```python
from build123d import *

# Parameters (mm, degrees)
SKETCH_W        = 232
SKETCH_H        = 132
PAD_DEPTH       = 140
SKETCH001_W     = 200
SKETCH001_H     = 100
POCKET_DEPTH    = 130
SKETCH002_W     = 216
SKETCH002_H     = 116
SKETCH002_W_2   = 200
SKETCH002_H_2   = 100
PAD001_DEPTH    = 8
FILLET_R        = 5
SKETCH008_R     = 3.5
POCKET003_DEPTH = 16


with BuildPart() as part:
    # Sketch → Pad (new body)
    with BuildSketch(Plane.XY):
        Rectangle(SKETCH_W, SKETCH_H)
    extrude(amount=PAD_DEPTH)

    # Sketch001 (on Face6 of Pad) → Pocket (cut)
    with BuildSketch(Plane.XY.offset(140)):
        Rectangle(SKETCH001_W, SKETCH001_H)
    extrude(amount=-POCKET_DEPTH, mode=Mode.SUBTRACT)

    # Sketch002 (on Face5 of Pocket) → Pad001 (join)
    with BuildSketch(Plane.XY.offset(140)):
        Rectangle(SKETCH002_W, SKETCH002_H)
        Rectangle(SKETCH002_W_2, SKETCH002_H_2, mode=Mode.SUBTRACT)
    extrude(amount=PAD001_DEPTH)

    # Fillet
    fillet_edges = [part.edges().sort_by_distance(p)[0] for p in [
        (-116, -66, 70),
        (116, -66, 70),
        (116, 66, 70),
        (0, -66, 0),
        (116, 0, 0),
        (-100, 50, 79),
        (-100, -50, 79),
        (-116, 66, 70),
        (100, -50, 79),
        (100, 50, 79),
        (100, 0, 10),
        (0, -50, 10),
        (0, 50, 10),
        (-100, 0, 10),
        (108, -58, 144),
        (108, 58, 144),
        (-108, -58, 144),
        (-108, 58, 144),
        (0, 66, 0),
        (-116, 0, 0),
    ]]
    fillet(fillet_edges, radius=FILLET_R)

    # Sketch008 (on Face10 of Fillet) → Pocket003 (cut)
    with BuildSketch(Plane.YZ.offset(116)):
        with Locations((25, 19.8)):
            Circle(SKETCH008_R)
    extrude(amount=-POCKET003_DEPTH, mode=Mode.SUBTRACT)


solid = part.part
```
CAD build for the part. Positions are in the model's coordinates, mm. A direction names the side the tool comes from. Coordinates: 2 decimals unless noted, no trailing zeros. Write each loop counter-clockwise with the first axis right and the second up, starting at its lowest first coordinate (ties: lowest second). Pieces come first, ordered by that corner, then holes. Notation, with made-up numbers: (53, 6) -> (68, 6) arc R12 ccw to (68, 15) -> close; hole circle Ø5 at (81.5, 7.5). An arc over 180 degrees is marked (long way). Return JSON: item names as keys, results as strings. Group by question number.
Q1. Cut at A-A, the plane y = 25. Give the cut face in (x, z).
Q2. Cut at C-C, the plane z = 84. Give the cut face in (x, y).
Q3. Flat gauge pins, fed straight in: pin 1 (6 mm diameter, centred on x = 18, y = 26.5, fed in from +Z); pin 2 (4 mm diameter, centred on y = 12, z = 142.5, fed in from +X). Where does each tip first touch, or does it go through?
Q4. Cut at D-D, the plane z = 19.8. Give the cut face in (x, y), then the cut area to 3 significant figures.
Q5. Which spindle directions (+Z, -Z, +X, -X, +Y, -Y) get a long thin tool onto all of the face, cutting with end or side? Do faces 4 (the face through (107, -56, 144)), 5 (the face through (-108, -1, 144)), 6 (the face through (-1, 58, 144)), 7 (the face through (-107, -56, 144)), 8 (the face through (1, -48, 11)). Say none if no direction does.
Q6. Drill centre lines: line 1 (X direction, y = -12.5, z = 110); line 2 (Y direction, x = 91.5, z = 66); line 3 (Z direction, x = 105.5, y = 25). Where is each one in solid material? Low to high.
Q7. Pull direction X, two halves, no side cores. Call faces 1 (the face through (107, 56, 144)), 2 (the face through (98, 49, 81)), 3 (the face through (-107, 56, 144)): released by +X, released by -X, zero draft, split by the parting line, or undercut.
Q8. Cut at B-B, the plane x = 82. Give the cut face in (y, z), then the cut area to 3 significant figures.
Returned:
{
 "1": {"outline": "(-116, 5) arc R5 ccw to (-111, 0) -> (111, 0) arc R5 ccw to (116, 5) -> (116, 16.3) -> (100, 16.3) -> (100, 15) arc R5 cw to (95, 10) -> (-95, 10) arc R5 cw to (-100, 15) -> (-100, 148) -> (-108, 148) -> (-108, 140) -> (-116, 140) -> close; (100, 23.3) -> (116, 23.3) -> (116, 140) -> (108, 140) -> (108, 148) -> (100, 148) -> close"},
 "2": {"outline": "(-116, -61) arc R5 ccw to (-111, -66) -> (111, -66) arc R5 ccw to (116, -61) -> (116, 61) arc R5 ccw to (111, 66) -> (-111, 66) arc R5 ccw to (-116, 61) -> close; hole (-100, -45) arc R5 ccw to (-95, -50) -> (95, -50) arc R5 ccw to (100, -45) -> (100, 45) arc R5 ccw to (95, 50) -> (-95, 50) arc R5 ccw to (-100, 45) -> close"},
 "3": {"pin 1": "stops at z = 10", "pin 2": "stops at x = 108"},
 "4": {"outline": "(-116, -61) arc R5 ccw to (-111, -66) -> (111, -66) arc R5 ccw to (116, -61) -> (116, 21.5) -> (100, 21.5) -> (100, -45) arc R5 cw to (95, -50) -> (-95, -50) arc R5 cw to (-100, -45) -> (-100, 45) arc R5 cw to (-95, 50) -> (95, 50) arc R5 cw to (100, 45) -> (100, 28.5) -> (116, 28.5) -> (116, 61) arc R5 ccw to (111, 66) -> (-111, 66) arc R5 ccw to (-116, 61) -> close", "area": "10,500 mm2"},
 "5": {"face 4": "+Z, +X, -Y", "face 5": "+Z, -X, +Y, -Y", "face 6": "+Z, +X, -X, +Y", "face 7": "+Z, -X, -Y", "face 8": "+Z"},
 "6": {"line 1": "x = -116 to -100, 100 to 116", "line 2": "y = -66 to -50, 50 to 66", "line 3": "z = 0 to 16.3, 23.3 to 148"},
 "7": {"face 1": "released by +X", "face 2": "undercut", "face 3": "released by -X"},
 "8": {"outline": "(-66, 5) arc R5 ccw to (-61, 0) -> (61, 0) arc R5 ccw to (66, 5) -> (66, 140) -> (58, 140) -> (58, 148) -> (50, 148) -> (50, 15) arc R5 cw to (45, 10) -> (-45, 10) arc R5 cw to (-50, 15) -> (-50, 148) -> (-58, 148) -> (-58, 140) -> (-66, 140) -> close", "area": "5,610 mm2"}
}
